For this review, use the dimensioned drawing (mm, ordinates from the lowest corner) and the shaded views. A direction names the side the tool comes from. Round coordinates to 2 decimals unless told otherwise and drop trailing zeros. Write each loop counter-clockwise with the first axis right and the second up, starting at its lowest first coordinate (ties: lowest second). Pieces come first, ordered by that corner, then holes. Notation, with made-up numbers: M 73.25,-34.5 L 105.25,-34.5 A29 cw 105.25,2.5 Z; hole C 68.25,-11 d10. An arc over 180 degrees is marked long. Use one line per item in the form item = value. Start each with the question number.
Item 1: For the marked faces 1 and 2, list the 3-axis set-ups (+Z, -Z, +X, -X, +Y, -Y) from which the entire face can be reached by the end or side of a thin tool; tool diameter is ignored.
Item 2: Add section C-C (z = 18.5). State the section outline as (x, y) points, and give its area (3 significant figures).
Item 3: For P1, Ø1.6, axis at y = 5, z = 16.5, coming from the -X side; P2, Ø1.5, axis at x = 39, y = 4.5, coming from the -Z side; P3, Ø3, axis at x = 71.45, z = 3.9, coming from the +Y side; P4, Ø1.5, axis at y = 3.5, z = 13.5, coming from the +X side, all flat-tipped, find the tip position at first contact; note any pin that passes through.
Item 4: Add section A-A (x = 71.45). State the section outline as (y, z) points.
Item 5: For line 1 (X direction, y = 0.55, z = 40.6); line 2 (X direction, y = 0.5, z = 40); line 3 (X direction, y = 5.75, z = 19.5), list the stretches that pass through material, from the lowest coordinate up. Write a range as [from, to].
Item 6: Add section D-D (y = 4.5). State the section outline as (x, z) points.
Item 7: Add section B-B (z = 40.6). State the section outline as (x, y) points.
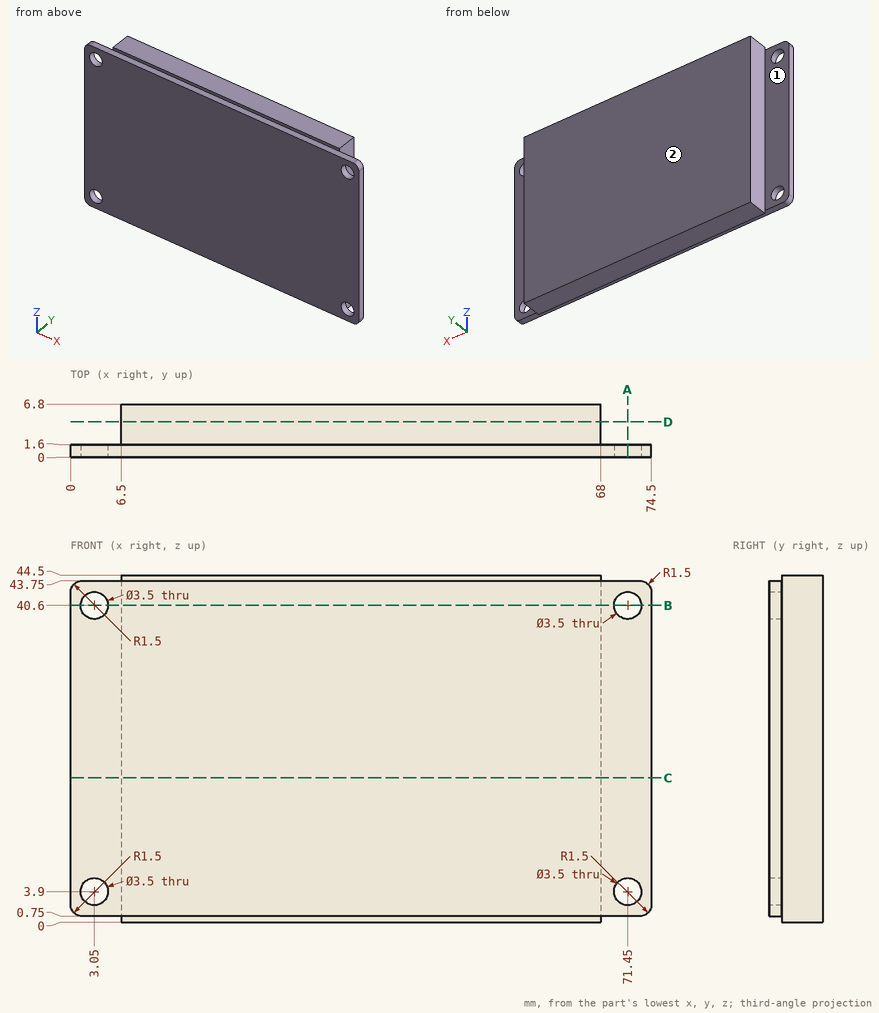
Calculated:
q1.face_1 = +Z, -Z, -X, +Y
q1.face_2 = +Z, -Z, +X, -X, +Y
q2.outline = M 0,0 L 74.5,0 L 74.5,1.6 L 68,1.6 L 68,6.8 L 6.5,6.8 L 6.5,1.6 L 0,1.6 Z
q2.area = 439 mm^2
q3.P1 = 6.5
q3.P2 = 0
q3.P3 = through
q3.P4 = 68
q4.outline = M 0,0.75 L 1.6,0.75 L 1.6,2.15 L 0,2.15 Z; M 0,5.65 L 1.6,5.65 L 1.6,38.85 L 0,38.85 Z; M 0,42.35 L 1.6,42.35 L 1.6,43.75 L 0,43.75 Z
q5.line_1 = [0, 1.3], [4.8, 69.7], [73.2, 74.5]
q5.line_2 = [0, 1.41], [4.69, 69.81], [73.09, 74.5]
q5.line_3 = [6.5, 68]
q6.outline = M 6.5,0 L 68,0 L 68,44.5 L 6.5,44.5 Z
q7.outline = M 0,0 L 1.3,0 L 1.3,1.6 L 0,1.6 Z; M 4.8,0 L 69.7,0 L 69.7,1.6 L 68,1.6 L 68,6.8 L 6.5,6.8 L 6.5,1.6 L 4.8,1.6 Z; M 73.2,0 L 74.5,0 L 74.5,1.6 L 73.2,1.6 Z
